Could you check a few things on this drawing? It's one solid part, dimensions in mm from its lowest x, y, z. A direction names the side the tool comes from. Round coordinates to 2 decimals unless told otherwise and drop trailing zeros. Write each loop counter-clockwise with the first axis right and the second up, starting at its lowest first coordinate (ties: lowest second). Pieces come first, ordered by that corner, then holes. Notation, with made-up numbers: M -39,89.5 L -6,89.5 A16 ccw -6,104.5 Z; hole C 1,64.25 d9. An arc over 180 degrees is marked long. One line per question, with ' | ' between items. Start each with the question number.
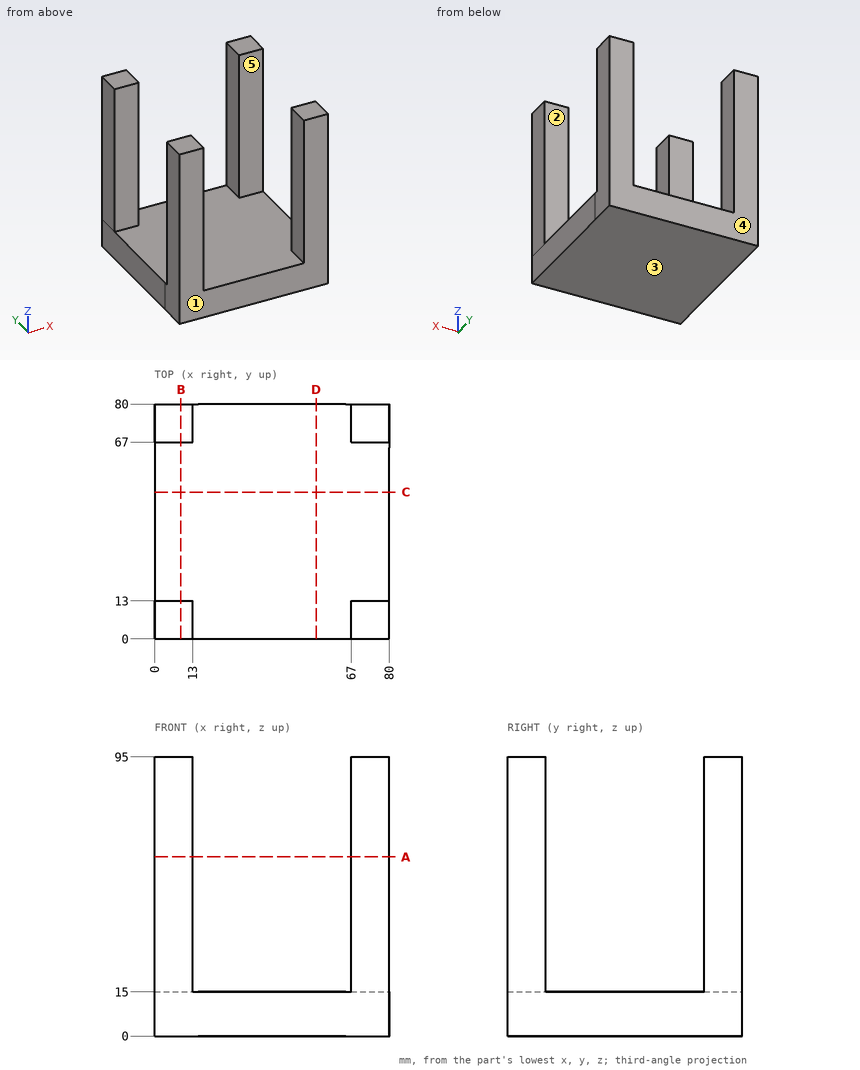
1. Suppose I cut it at A-A (z = 61). Write out the boundary of the cut face in (x, y).
2. Suppose I cut it at C-C (y = 50). Write out the boundary of the cut face in (x, z).
3. Which directions (+Z, -Z, +X, -X, +Y, -Y) give clear straight access to the entire face, cutting with the end or side of a thin tool? Please do the marked faces 1 and 2.
4. Suppose I cut it at B-B (x = 9). Write out the boundary of the cut face in (y, z), and give its area (3 significant figures).
5. If we mould it in two halves opening along Y, with no side actions, what happens to the marked faces 3, 4 and 5? For each: released by +Y, released by -Y, zero draft, split by the parting line, or undercut.
6. I'm going to push flat-ended pins straight in: P1, Ø12, axis at x = 17.5, y = 11, coming from the +Z side; P2, Ø1, axis at x = 38.5, y = 34.5, coming from the +Z side. Where does each tip first touch, or does it pass through?
7. I need wall thicknesses on line 1 along X through (y, z) = (70.5, 44.5); line 2 along Z through (x, y) = (26, 22). Which ranges of each line are inside material? Lowest first, please. Write a range as from..to.
Computed:
1) outline: M 0,0 L 13,0 L 13,13 L 0,13 Z; M 0,67 L 13,67 L 13,80 L 0,80 Z; M 67,0 L 80,0 L 80,13 L 67,13 Z; M 67,67 L 80,67 L 80,80 L 67,80 Z
2) outline: M 0,0 L 80,0 L 80,15 L 0,15 Z
3) face 1: +Z, -Z, +X, -X, -Y | face 2: +Z, +X, -X
4) outline: M 0,0 L 80,0 L 80,95 L 67,95 L 67,15 L 13,15 L 13,95 L 0,95 Z | area: 3,280 mm²
5) face 3: zero draft | face 4: released by +Y | face 5: undercut
6) P1: stops at z = 95 | P2: stops at z = 15
7) line 1: x = 0..13, 67..80 | line 2: z = 0..15
